```python
from build123d import *

# Parameters (mm, degrees)
BOSS_EXTRU_1_DEPTH           = 200
BOSS_EXTRU_1_DEPTH_BACK      = 200
ESQUISSE1_R                  = 25
ESQUISSE2_R                  = 24
ENL_V_MAT_EXTRU_1_DEPTH      = 400
ENL_V_MAT_EXTRU_2_DEPTH      = 60
ENL_V_MAT_EXTRU_2_DEPTH_BACK = 180
ESQUISSE3_W                  = 240
ESQUISSE3_H                  = 600


with BuildPart() as part:
    # Esquisse1 → Boss.-Extru.1 (new, two sides: drawn at the far end of the back side and taken through both)
    with BuildSketch(Plane(origin=(0, 0, 0), x_dir=(1, 0, 0), z_dir=(0, 1, 0)).offset(-BOSS_EXTRU_1_DEPTH_BACK)):
        with Locations(Location((0, 0, 0), (0, 0, 270))):
            Circle(ESQUISSE1_R)
    extrude(amount=BOSS_EXTRU_1_DEPTH + BOSS_EXTRU_1_DEPTH_BACK)

    # Esquisse2 → Enl_v. mat.-Extru.1 (cut)
    with BuildSketch(Plane(origin=(0, 200, 0), x_dir=(1, 0, 0), z_dir=(0, 1, 0))):
        with Locations(Location((0, 0, 0), (0, 0, 270))):
            Circle(ESQUISSE2_R)
    extrude(amount=-ENL_V_MAT_EXTRU_1_DEPTH, mode=Mode.SUBTRACT)

    # Esquisse3 → Enl_v. mat.-Extru.2 (cut, two sides: drawn at the far end of the back side and taken through both)
    with BuildSketch(Plane(origin=(0, 0, 0), x_dir=(1, 0, 0), z_dir=(0, 1, 0)).offset(-ENL_V_MAT_EXTRU_2_DEPTH_BACK)):
        with Locations((-120, 0)):
            Rectangle(ESQUISSE3_W, ESQUISSE3_H)
    extrude(amount=ENL_V_MAT_EXTRU_2_DEPTH + ENL_V_MAT_EXTRU_2_DEPTH_BACK, mode=Mode.SUBTRACT)


solid = part.part
```
Verification items for the finished model (mm, model axes). A direction names the side the tool comes from. Coordinates: 2 decimals unless noted, no trailing zeros. Loops run counter-clockwise (first coordinate to the right, second up) from the corner with the lowest first, then second, coordinate; pieces in that order, holes last. Notation, with made-up numbers: (66, 27.5) -> (111, 27.5) arc R25 cw to (111, 45.5) -> close; hole circle Ø2 at (40.5, -18.75). An arc over 180 degrees is marked (long way). Put each result on its own line as item: value.
1. Gauge pin test, flat ends, axial feed: P1, Ø0.5, axis at y = -78.5, z = 24.5, coming from the -X side; P2, Ø1, axis at y = -45.5, z = 12, coming from the +X side; P3, Ø1, axis at x = -2, y = -140, coming from the +Z side; P4, Ø10, axis at y = 40, z = 14.5, coming from the -X side. Record the tip position at first contact, or that the pin passes through.
Result set:
P1: stops at x = 0
P2: stops at x = 22.2
P3: passes through
P4: stops at x = 13.99
2. Tool access check on faces 1 (the face through (-24.6, -180, -0.1)), 2 (the face through (9.4, -200, -22.3)). Record the directions out of +Z, -Z, +X, -X, +Y, -Y that give a thin tool (end or side, any length) a straight path to the whole face; none if there is none.
Result set:
face 1: +Z, -Z, -X
face 2: +Z, -Z, +X, -X, -Y
3. Section check D-D, the plane y = -126. Record the boundary of the cut face in (x, z), then the cut area to 3 significant figures.
Result set:
outline: (0, -25) arc R25 ccw to (0, 25) -> (0, 24) arc R24 cw to (0, -24) -> close
area: 77.0 mm^2
4. Section check C-C, the plane x = 14.5. Record the boundary of the cut face in (y, z).
Result set:
outline: (-200, -20.37) -> (200, -20.37) -> (200, -19.12) -> (-200, -19.12) -> close; (-200, 19.12) -> (200, 19.12) -> (200, 20.37) -> (-200, 20.37) -> close
5. Section check A-A, the plane z = 0. Record the boundary of the cut face in (x, y), then the cut area to 3 significant figures.
Result set:
outline: (-25, -200) -> (-24, -200) -> (-24, -180) -> (-25, -180) -> close; (-25, 60) -> (-24, 60) -> (-24, 200) -> (-25, 200) -> close; (24, -200) -> (25, -200) -> (25, 200) -> (24, 200) -> close
area: 560 mm^2
6. Mould release check, pull along Z, two halves, no side actions. Record for faces 3 (the face through (23.8, 47.2, -3.1)), 4 (the face through (9.4, 200, -22.3)), 5 (the face through (24.787, -2.8, -3.255)): pulls with the +Z half, pulls with the -Z half, needs draft (parallel to the pull), parting line crosses it, or undercut.
Result set:
face 3: undercut
face 4: needs draft
face 5: parting line crosses it
7. Section check B-B, the plane x = -4.5. Record the boundary of the cut face in (y, z), then the cut area to 3 significant figures.
Result set:
outline: (-200, -24.59) -> (-180, -24.59) -> (-180, -23.57) -> (-200, -23.57) -> close; (-200, 23.57) -> (-180, 23.57) -> (-180, 24.59) -> (-200, 24.59) -> close; (60, -24.59) -> (200, -24.59) -> (200, -23.57) -> (60, -23.57) -> close; (60, 23.57) -> (200, 23.57) -> (200, 24.59) -> (60, 24.59) -> close
area: 326 mm^2
8. Thickness scan on line 1 (Z direction, x = 0, y = 88); line 2 (Z direction, x = 20, y = 53.5). Record the ranges inside material, lowest first.
Result set:
line 1: z = -25 to -24, 24 to 25
line 2: z = -15 to -13.27, 13.27 to 15
